from build123d import *

# Parameters (mm, degrees)
SKETCH_1_W      = 32
SKETCH_1_H      = 13
EXTRUDE_1_DEPTH = 23
SKETCH_2_R      = 1.5
EXTRUDE_2_DEPTH = 7
SKETCH_3_W      = 9.5
SKETCH_3_H      = 1
EXTRUDE_3_DEPTH = 1


with BuildPart() as part:
    # 草图1 → 凸台-拉伸1 (new body)
    with BuildSketch(Plane.XY):
        with Locations((16, 6.5)):
            Rectangle(SKETCH_1_W, SKETCH_1_H)
    extrude(amount=EXTRUDE_1_DEPTH)

    # 草图2 → 凸台-拉伸2 (add)
    with BuildSketch(Plane.XY.offset(23)):
        with Locations((27.678688567, 6.5)):
            Circle(SKETCH_2_R)
    extrude(amount=EXTRUDE_2_DEPTH)

    # 草图3 → 凸台-拉伸3 (add)
    with BuildSketch(Plane.XY.offset(30)):
        with Locations((22.928688567, 6.5)):
            Rectangle(SKETCH_3_W, SKETCH_3_H)
    extrude_3 = extrude(amount=EXTRUDE_3_DEPTH)

    # 镜向1: 凸台-拉伸3 across plane
    add(extrude_3.mirror(Plane(origin=(27.678688567, 7, 31), x_dir=(0, 0, 1), z_dir=(-1, 0, 0))))


solid = part.part
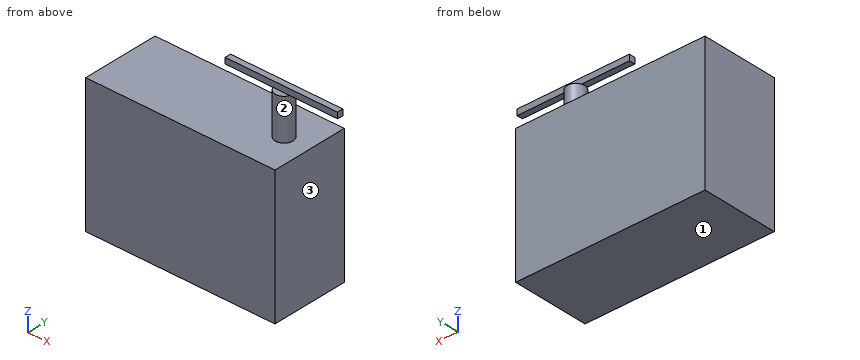
Design review of the part built by this model. Coordinates are the model's own, in mm. Face numbers are marked on the shaded views. Give positions to 0.01 mm unless a question says otherwise; leave off trailing zeros. Loops run counter-clockwise (first coordinate to the right, second up) from the corner with the lowest first, then second, coordinate; pieces in that order, holes last. Notation, with made-up numbers: M 78.25,74.5 L 134.25,74.5 A20 ccw 134.25,105.5 Z; hole C 4,54 d4. An arc over 180 degrees is marked long. One line per question, with ' | ' between items. Start each with the question number.
1. Add section B-B (y = 6.5). Write out the cut boundary in (x, z).
2. Insertion check: P1, Ø0.8, axis at x = 29, z = 30.5, coming from the -Y side; P2, Ø0.5, axis at y = 6.5, z = 30.5, coming from the -X side; P3, Ø0.8, axis at x = 34.5, y = 6.5, coming from the -Z side. Each pin has a flat end and moves straight along its axis. Give the tip position at first contact, or say it passes through.
3. To check wall thickness, follow L1, parallel to Z at x = 21, y = 6.5; L2, parallel to Z at x = 17, y = 8.25; L3, parallel to X at y = 3.25, z = 13. State the ranges of each line that lie inside material, in increasing order.
4. Add section A-A (x = 21.5). Write out the cut boundary in (y, z).
5. Add section C-C (z = 9.5). Write out the cut boundary in (x, y).
6. Add section D-D (x = 12.5). Write out the cut boundary in (y, z), plus the area to 3 significant figures.
7. The part is to be moulded in two halves that separate along Z. For the marked faces 1, 2 and 3, say which applies: released by +Z, released by -Z, zero draft, split by the parting line, or undercut.
Worked out:
1) outline: M 0,0 L 32,0 L 32,23 L 29.18,23 L 29.18,30 L 37.18,30 L 37.18,31 L 18.18,31 L 18.18,30 L 26.18,30 L 26.18,23 L 0,23 Z
2) P1: stops at y = 6 | P2: stops at x = 18.18 | P3: stops at z = 30
3) L1: z = 0 to 23, 30 to 31 | L2: z = 0 to 23 | L3: x = 0 to 32
4) outline: M 0,0 L 13,0 L 13,23 L 0,23 Z; M 6,30 L 7,30 L 7,31 L 6,31 Z
5) outline: M 0,0 L 32,0 L 32,13 L 0,13 Z
6) outline: M 0,0 L 13,0 L 13,23 L 0,23 Z | area: 299 mm²
7) face 1: released by -Z | face 2: undercut | face 3: zero draft
